Here's the drawing with two shaded views (mm, measured from the low corner). I have some questions. A direction names the side the tool comes from. Round coordinates to 2 decimals unless told otherwise and drop trailing zeros. Loops run counter-clockwise (first coordinate to the right, second up) from the corner with the lowest first, then second, coordinate; pieces in that order, holes last. Notation, with made-up numbers: (17.5, 79.5) -> (35.5, 79.5) arc R22 cw to (35.5, 106.5) -> close; hole circle Ø2 at (29.5, 53). An arc over 180 degrees is marked (long way). Write each question's results on one line, items separated by ' | '. Start each with the question number.
1) If I drill on probe 1 along Y at (x, z) = (56, 19); probe 2 along X at (y, z) = (7, 6); probe 3 along X at (y, z) = (15, 21), over which ranges is the centre line in solid material (lowest first)?
2) Imagine slicing it at D-D, the plane z = 15. Give the number of separate pieces and of enclosed holes in the cut face, plus the area to 3 significant figures.
3) Imagine slicing it at A-A, the plane x = 12.7. List the corners of the cut face in (y, z) for me.
4) For P1, Ø3, axis at x = 30.96, z = 15.88, coming from the -Y side; P2, Ø1, axis at y = 11, z = 15.5, coming from the +X side, each with a flat end and sliding along its axis, tell me the tip position at first contact or that it passes through.
5) Which directions (+Z, -Z, +X, -X, +Y, -Y) give clear straight access to the entire face, cutting with the end or side of a thin tool? Please do the marked faces 5 and 6.
6) We'd pull the mould along Y, two halves only. Please class the marked faces 1, 2, 3 and 4: pulls with the +Y half, pulls with the -Y half, needs draft (parallel to the pull), parting line crosses it, or undercut.
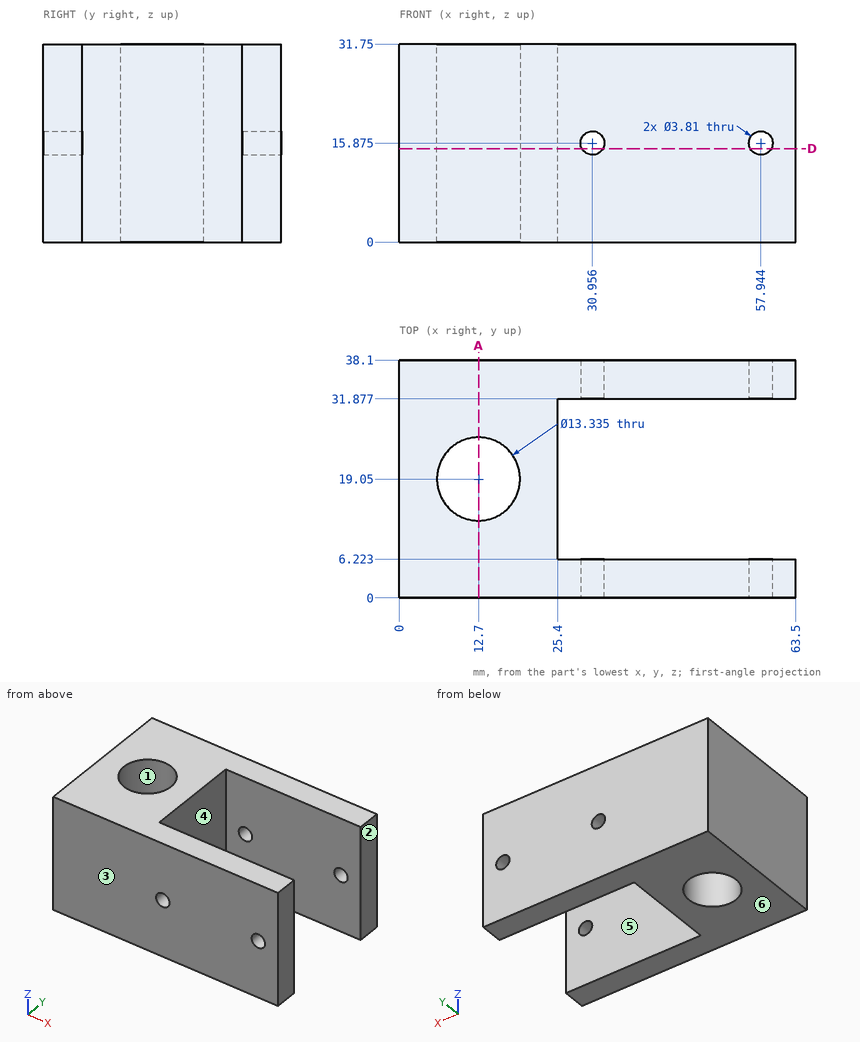
Checked values:
1) probe 1: 0 to 6.22, 31.88 to 38.1 | probe 2: 0 to 25.4 | probe 3: 0 to 7.4, 18 to 25.4
2) separate pieces: 5 | enclosed holes: 1 | area: 1,220 mm^2
3) outline: (0, 0) -> (12.38, 0) -> (12.38, 31.75) -> (0, 31.75) -> close; (25.72, 0) -> (38.1, 0) -> (38.1, 31.75) -> (25.72, 31.75) -> close
4) P1: through | P2: x = 25.4
5) face 5: +Z, -Z, +X | face 6: -Z, +X, -X, +Y, -Y
6) face 1: undercut | face 2: needs draft | face 3: pulls with the -Y half | face 4: undercut
